Build history of the part. All positions in model axes, mm. Give positions to 0.01 mm unless a question says otherwise; leave off trailing zeros. Loops run counter-clockwise (first coordinate to the right, second up) from the corner with the lowest first, then second, coordinate; pieces in that order, holes last. Notation, with made-up numbers: (59.5, 41) - (64.5, 41) arc R22 cw to (64.5, 50) - close; hole circle Ø1 at (23, -4.75). An arc over 180 degrees is marked (long way). Return JSON: item names as keys, results as strings. Group by question number.
1) Slice it at D-D (y = 26). List the corners of the cut face in (x, z), and give its area (3 significant figures).
2) Drop flat-ended pins along their axis: pin 1 (5 mm diameter, centred on y = 14.5, z = -4.5, fed in from +X); pin 2 (1.5 mm diameter, centred on x = 0.5, z = 1, fed in from +Y); pin 3 (8 mm diameter, centred on y = 9.5, z = 0.5, fed in from -X). Give the stop position or say it passes through.
3) Slice it at A-A (x = 0). List the corners of the cut face in (y, z), and give its area (3 significant figures).
4) Drill centre lines: probe 1 along Y at (x, z) = (19.5, 5); probe 2 along X at (y, z) = (11, 8.5); probe 3 along X at (y, z) = (4, 15.5). Where is each one in solid material? Low to high. Write a range as from..to.
5) Slice it at B-B (z = -1.5). List the corners of the cut face in (x, y), and give its area (3 significant figures).
6) Slice it at C-C (y = 30.5). List the corners of the cut face in (x, z), and give its area (3 significant figures).
```python
from build123d import *

# Parameters (mm, degrees)
BOSS_EXTRUDE1_DEPTH     = 7
SKETCH2_R               = 11.5
BOSS_EXTRUDE2_DEPTH     = 26
CUT_EXTRUDE1_DEPTH      = 26
CUT_EXTRUDE1_DEPTH_BACK = 26


with BuildPart() as part:
    # Sketch1 → Boss-Extrude1 (new body)
    with BuildSketch(Plane(origin=(0, 0, 0), x_dir=(1, 0, 0), z_dir=(0, 1, 0))):
        with BuildLine():
            Line((24.778235728, 3.32250421), (10.896730509, 3.67576716))
            ThreePointArc((10.896730509, 3.67576716), (-4.207828527, 10.702531433), (-10.482370924, -4.729682845))
            Line((-10.482370924, -4.729682845), (-20.036775025, -14.950841))
            ThreePointArc((-20.036775025, -14.950841), (9.439234539, -23.149532421), (24.778235728, 3.32250421))
        make_face()
    extrude(amount=BOSS_EXTRUDE1_DEPTH)

    # Sketch2 → Boss-Extrude2 (add)
    with BuildSketch(Plane(origin=(0, 7, 0), x_dir=(1, 0, 0), z_dir=(0, 1, 0))):
        Circle(SKETCH2_R)
    extrude(amount=BOSS_EXTRUDE2_DEPTH)

    # Sketch5 → Cut-Extrude1 (cut, two sides)
    with BuildSketch(Plane(origin=(0, 0, 0), x_dir=(0, 0, -1), z_dir=(1, 0, 0))) as cut_extrude1_sk:
        Polygon((11.5, 33), (11.5, 9.182802783), (-11.5, 33), align=None)
    extrude(amount=CUT_EXTRUDE1_DEPTH, mode=Mode.SUBTRACT)
    extrude(cut_extrude1_sk.sketch, amount=-CUT_EXTRUDE1_DEPTH_BACK, mode=Mode.SUBTRACT)


solid = part.part
```
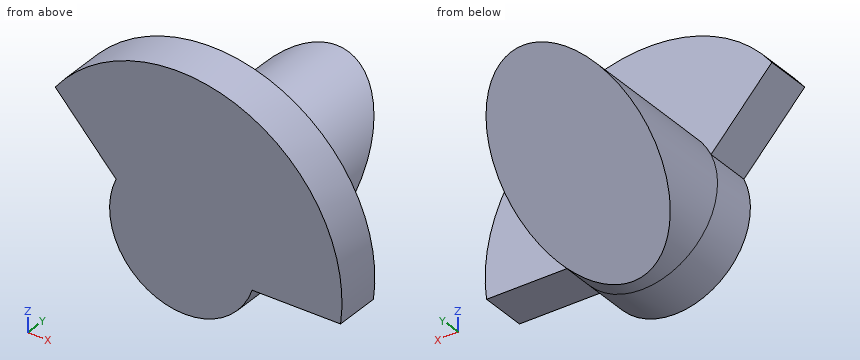
Results:
{
 "1": {"outline": "(-10.48, 4.74) - (10.48, 4.74) arc R11.5 ccw to start", "area": "102 mm2"},
 "2": {"pin 1": "x = 11.32", "pin 2": "y = 22.9", "pin 3": "x = -11.5"},
 "3": {"outline": "(0, -11.5) - (9.18, -11.5) - (33, 11.5) - (7, 11.5) - (7, 25) - (0, 25) - close", "area": "580 mm2"},
 "4": {"probe 1": "0..7", "probe 2": "-7.75..7.75", "probe 3": "-19.62..19.62"},
 "5": {"outline": "(-11.4, 0) - (24.95, 0) - (24.95, 7) - (11.4, 7) - (11.4, 19.54) - (-11.4, 19.54) - close", "area": "540 mm2"},
 "6": {"outline": "(-7.05, 9.09) - (7.05, 9.09) arc R11.5 ccw to start", "area": "23.2 mm2"}
}
